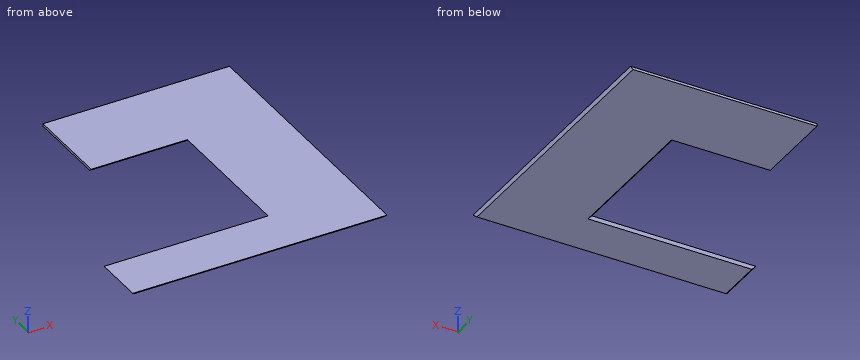
```python
from build123d import *

# Parameters (mm, degrees)
F1_DEPTH = 19.05
F2_SIZE  = 19.04999


# Not quite as in the source:
# - a fillet or chamfer is up to 0.001 mm smaller than in the source, because OpenCascade refuses the exact size


with BuildPart() as f1:
    # F0 (on Top) → F1 (new body)
    with BuildSketch(Plane.XY):
        Polygon((1244.6, 0), (0, 0), (0, -381), (1930.4, -381), (1930.4, 1714.5), (514.35, 1714.5), (514.35, 1073.15), (1244.6, 1073.15), align=None)
    extrude(amount=F1_DEPTH)

    # F2 (size 19.05 in the source; OpenCascade refuses exactly that, so slightly less here)
    f2_edges = [f1.edges().sort_by_distance(p)[0] for p in [
        (965.2, -381, 0),
        (1930.4, 666.75, 0),
        (879.475, 1073.15, 0),
        (1244.6, 536.575, 0),
        (622.3, 0, 0),
        (0, -190.5, 0),
    ]]
    chamfer(f2_edges, length=F2_SIZE)


solid = f1.part
```
The listing builds one solid part. Answer for the finished solid, in the listing's coordinates (mm). Give positions to 0.01 mm unless a question says otherwise; leave off trailing zeros. Write each loop counter-clockwise with the first axis right and the second up, starting at its lowest first coordinate (ties: lowest second). Pieces come first, ordered by that corner, then holes. Notation, with made-up numbers: (59, 13.25) -> (89, 13.25) arc R25 ccw to (89, 42.25) -> close; hole circle Ø2 at (-25, 31.25). An arc over 180 degrees is marked (long way). Write item = value, one per line. Start each with the question number.
1) The part is cut by section D-D, the plane z = 7. Determine the outline of the cut face in (x, y).
2) Each of these flat-tipped pins is pushed along its axis until it touches: pin 1 (9.5 mm diameter, centred on y = 1334.5, z = 9.5, fed in from -X); pin 2 (5 mm diameter, centred on y = 291.5, z = 8, fed in from +X); pin 3 (1 mm diameter, centred on y = 560.5, z = 8.5, fed in from -X). Where does it stop, or does it pass through?
3) Straight lines are drawn through the part: line 1 along Y through (x, z) = (1002, 13); line 2 along Y through (x, z) = (1223, 7); line 3 along X through (y, z) = (-98, 16). For each, find the intervals that lie inside material, in ascending order.
Solutions:
q1.outline = (12.05, -368.95) -> (1918.35, -368.95) -> (1918.35, 1714.5) -> (514.35, 1714.5) -> (514.35, 1085.2) -> (1256.65, 1085.2) -> (1256.65, -12.05) -> (12.05, -12.05) -> close
q2.pin_1 = 514.35
q2.pin_2 = 1921.85
q2.pin_3 = 1254.65
q3.line_1 = -374.95 to -6.05, 1079.2 to 1714.5
q3.line_2 = -368.95 to -12.05, 1085.2 to 1714.5
q3.line_3 = 3.05 to 1927.35
